from build123d import *

# Parameters (mm, degrees)
BOSS_EXTRUDE1_DEPTH = 50.8
BOSS_EXTRUDE3_START = 4.5
BOSS_EXTRUDE3_DEPTH = 4.5
BOSS_EXTRUDE4_DEPTH = 5
SKETCH6_R           = 1.75
CUT_EXTRUDE1_DEPTH  = 18.75
SKETCH7_W           = 101.6
SKETCH7_H           = 0.5
CUT_EXTRUDE2_DEPTH  = 5.461
SKETCH8_W           = 124.6
SKETCH8_H           = 0.9
CUT_EXTRUDE3_DEPTH  = 10.6
FILLET1_SIZE        = 0.5


with BuildPart() as part:
    # Sketch1 → Boss-Extrude1 (new, symmetric)
    with BuildSketch(Plane(origin=(0, 0, 0), x_dir=(0, 0, -1), z_dir=(1, 0, 0))):
        with BuildLine():
            Line((0, 0), (60, 0))
            ThreePointArc((60, 0), (64.685586675, -3.254927648), (63.270675103, -8.781888995))
            Line((63.270675103, -8.781888995), (0, -63.5))
            Line((0, -63.5), (0, -70.110453145))
            Line((0, -70.110453145), (66.541350207, -12.56377799))
            ThreePointArc((66.541350207, -12.56377799), (69.37117335, -1.509855296), (60, 5))
            Line((60, 5), (0, 5))
            Line((0, 5), (0, 0))
        make_face()
    extrude(amount=BOSS_EXTRUDE1_DEPTH, both=True)

    # Sketch3 → Boss-Extrude3 (add)
    with BuildSketch(Plane(origin=(50.8, 0, 0), x_dir=(0, 0, -1), z_dir=(1, 0, 0)).offset(BOSS_EXTRUDE3_START)):
        with BuildLine():
            Line((60, 5), (0, 5))
            Line((0, 5), (0, 0))
            Line((0, 0), (60, 0))
            ThreePointArc((60, 0), (64.685586675, -3.254927648), (63.270675103, -8.781888995))
            Line((63.270675103, -8.781888995), (0, -63.5))
            Line((0, -63.5), (0, -70.110453145))
            Line((0, -70.110453145), (66.541350207, -12.56377799))
            ThreePointArc((66.541350207, -12.56377799), (69.37117335, -1.509855296), (60, 5))
        make_face()
        with BuildLine():
            Line((0, 0), (0, -63.5))
            Line((0, -63.5), (63.270675103, -8.781888995))
            ThreePointArc((63.270675103, -8.781888995), (64.685586675, -3.254927648), (60, 0))
            Line((60, 0), (0, 0))
        make_face()
    boss_extrude3 = extrude(amount=-BOSS_EXTRUDE3_DEPTH)

    # Mirror1: Boss-Extrude3 across plane
    add(boss_extrude3.mirror(Plane(origin=(0, 0, 0), x_dir=(0, 0, 1), z_dir=(1, 0, 0))))

    # Sketch4 → Boss-Extrude4 (add)
    with BuildSketch(Plane.XY):
        Polygon((-50.8, 5), (-50.8, -63.5), (50.8, -63.5), (50.8, 5), (62.3, 5), (62.3, -70.110453145), (-62.3, -70.110453145), (-62.3, 5), align=None)
    extrude(amount=-BOSS_EXTRUDE4_DEPTH)

    # Sketch6 → Cut-Extrude1 (cut)
    with BuildSketch(Plane.XY):
        with Locations((-57.5, -2.146)):
            Circle(SKETCH6_R)
        with Locations((-57.5, -62.146)):
            Circle(SKETCH6_R)
        with Locations((57.5, -62.146)):
            Circle(SKETCH6_R)
        with Locations((57.5, -2.146)):
            Circle(SKETCH6_R)
    extrude(amount=-CUT_EXTRUDE1_DEPTH, mode=Mode.SUBTRACT)

    # Sketch7 → Cut-Extrude2 (cut)
    with BuildSketch(Plane.XY):
        with Locations((0, 0.25)):
            Rectangle(SKETCH7_W, SKETCH7_H)
    extrude(amount=-CUT_EXTRUDE2_DEPTH, mode=Mode.SUBTRACT)

    # Sketch8 → Cut-Extrude3 (cut)
    with BuildSketch(Plane.XY):
        with Locations((0, 4.55)):
            Rectangle(SKETCH8_W, SKETCH8_H)
    extrude(amount=-CUT_EXTRUDE3_DEPTH, mode=Mode.SUBTRACT)

    # Fillet1
    fillet1_edges = [part.edges().sort_by_distance(p)[0] for p in [
        (0, 0.5, 0),
        (0, 4.1, 0),
    ]]
    chamfer(fillet1_edges, length=FILLET1_SIZE)


solid = part.part
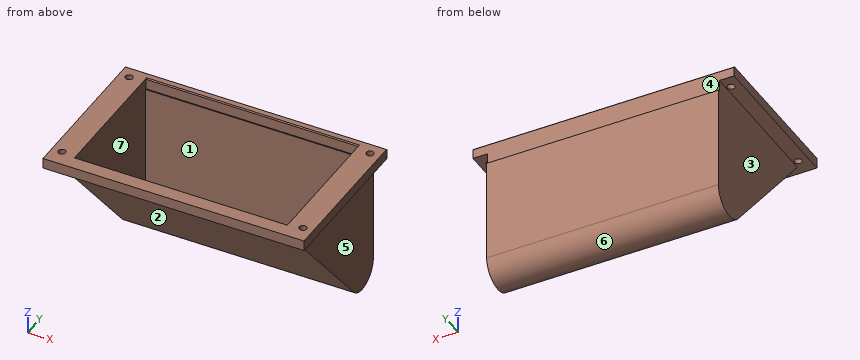
Can you work these out from the model? Positions are in its coordinate system, mm. Face numbers are marked on the shaded views. A direction names the side the tool comes from. Give positions to 0.01 mm unless a question says otherwise; leave off trailing zeros. Loops run counter-clockwise (first coordinate to the right, second up) from the corner with the lowest first, then second, coordinate; pieces in that order, holes last. Notation, with made-up numbers: (44.5, -9) -> (95.5, -9) arc R24 cw to (95.5, 3) -> close; hole circle Ø6 at (11.5, 70). An arc over 180 degrees is marked (long way). Use one line per item in the form item = value.
1) Will these pins go through, and if not, where does the flat tip stop? pin 1 (19.5 mm diameter, centred on y = -43.5, z = -26, fed in from -X); pin 2 (1.5 mm diameter, centred on x = 39, y = -11.5, fed in from -Z); pin 3 (0.6 mm diameter, centred on x = 19, y = 0.5, fed in from +Z); pin 4 (3 mm diameter, centred on x = -57.5, y = -2.146, fed in from -Z).
Answers:
pin_1 = -55.3
pin_2 = -68.18
pin_3 = -0.2
pin_4 = through
2) If we section it at A-A (x = -57.5): Please give me the cut outline in (y, z).
Answers:
outline = (-70.11, -5) -> (-63.9, -5) -> (-63.9, 0) -> (-70.11, 0) -> close; (-60.4, -5) -> (-3.9, -5) -> (-3.9, 0) -> (-60.4, 0) -> close; (-0.4, -5) -> (4.1, -5) -> (4.1, -0.5) -> (3.6, 0) -> (-0.4, 0) -> close
3) If we section it at D-D (x = -9.5): Please give me the cut outline in (y, z), plus the area to 3 significant figures.
Answers:
outline = (-70.11, -5) -> (-65.79, -5) -> (-12.56, -66.54) arc R10 ccw to (5, -60) -> (5, -10.6) -> (4.1, -10.6) -> (4.1, -0.5) -> (3.6, 0) -> (1, 0) -> (0.5, -0.5) -> (0.5, -5.46) -> (0, -5.46) -> (0, -60) arc R5 cw to (-8.78, -63.27) -> (-63.5, 0) -> (-70.11, 0) -> close
area = 818 mm²
4) If we section it at B-B (z = -31.5): Please give me the cut outline in (x, y), plus the area to 3 significant figures.
Answers:
outline = (-55.3, -42.87) -> (55.3, -42.87) -> (55.3, 5) -> (-55.3, 5) -> close; hole (-50.8, -36.26) -> (50.8, -36.26) -> (50.8, 0) -> (-50.8, 0) -> close
area = 1,610 mm²
5) I need wall thicknesses on line 1 along Y through (x, z) = (-57.5, -3.25); line 2 along X through (y, z) = (-7.5, -9); line 3 along Y through (x, z) = (-57, -3). Which ranges of each line are inside material? Lowest first, please.
Answers:
line_1 = -70.11 to -63.9, -60.4 to -3.9, -0.4 to 4.1
line_2 = -55.3 to -50.8, 50.8 to 55.3
line_3 = -70.11 to -63.82, -60.47 to -3.82, -0.47 to 4.1
6) If we section it at C-C (y = -34.5): Please give me the cut outline in (x, z), plus the area to 3 significant figures.
Answers:
outline = (-62.3, -5) -> (-55.3, -5) -> (-55.3, -41.18) -> (55.3, -41.18) -> (55.3, -5) -> (62.3, -5) -> (62.3, 0) -> (50.8, 0) -> (50.8, -33.53) -> (-50.8, -33.53) -> (-50.8, 0) -> (-62.3, 0) -> close
area = 1,220 mm²
7) For the marked faces 1, 2 and 3, which set-ups out of +Z, -Z, +X, -X, +Y, -Y let a thin tool reach every point of the face, with its end or its side?
Answers:
face_1 = +Z
face_2 = -Z, +X, -X, -Y
face_3 = -Z, -X, +Y, -Y
8) We'd pull the mould along Y, two halves only. Please class the marked faces 4, 5, 6 and 7: released by +Y, released by -Y, zero draft, split by the parting line, or undercut.
Answers:
face_4 = released by +Y
face_5 = zero draft
face_6 = split by the parting line
face_7 = undercut
